CAD build for the part. Positions are in the model's coordinates, mm. Coordinates: 2 decimals unless noted, no trailing zeros. Loops run counter-clockwise (first coordinate to the right, second up) from the corner with the lowest first, then second, coordinate; pieces in that order, holes last. Notation, with made-up numbers: (83.5, 76) - (109.5, 76) arc R22 cw to (109.5, 92) - close; hole circle Ø9 at (49.25, 30). An arc over 180 degrees is marked (long way). Put each result on its own line as item: value.
```python
from build123d import *

# Parameters (mm, degrees)
SKETCH_1_W          = 23.5
SKETCH_1_H          = 10
SKETCH_1_R          = 1.6
EXTRUDE_1_DEPTH     = 5
SKETCH_2_R          = 2
CUT_EXTRUDE_1_DEPTH = 10


with BuildPart() as part:
    # 草图1 → 凸台-拉伸1 (new body)
    with BuildSketch(Plane.XY):
        Rectangle(SKETCH_1_W, SKETCH_1_H)
        with Locations((-8.5, 0)):
            Circle(SKETCH_1_R, mode=Mode.SUBTRACT)
        with Locations((8.5, 0)):
            Circle(SKETCH_1_R, mode=Mode.SUBTRACT)
    extrude(amount=EXTRUDE_1_DEPTH)

    # 草图2 → 切除-拉伸1 (cut)
    with BuildSketch(Plane.XY.offset(5)):
        Circle(SKETCH_2_R)
    extrude(amount=-CUT_EXTRUDE_1_DEPTH, mode=Mode.SUBTRACT)


solid = part.part
```
Q1. Wall check: L1, parallel to X at y = -0.5, z = 2.15; L2, parallel to Y at x = 8.5, z = 1.4; L3, parallel to Y at x = 0, z = 1.6. Give the ranges that are in metal, low to high. Write a range as from..to.
Determined:
L1: -11.75..-10.02, -6.98..-1.94, 1.94..6.98, 10.02..11.75
L2: -5..-1.6, 1.6..5
L3: -5..-2, 2..5
Q2. Slice it at B-B, the plane z = 4. Give the cut face in (x, y), then the cut area to 3 significant figures.
Determined:
outline: (-11.75, -5) - (11.75, -5) - (11.75, 5) - (-11.75, 5) - close; hole circle Ø3.2 at (-8.5, 0); hole circle Ø4 at (0, 0); hole circle Ø3.2 at (8.5, 0)
area: 206 mm2
Q3. Slice it at C-C, the plane x = -8.5. Give the cut face in (y, z).
Determined:
outline: (-5, 0) - (-1.6, 0) - (-1.6, 5) - (-5, 5) - close; (1.6, 0) - (5, 0) - (5, 5) - (1.6, 5) - close
Q4. Slice it at A-A, the plane x = 0. Give the cut face in (y, z), then the cut area to 3 significant figures.
Determined:
outline: (-5, 0) - (-2, 0) - (-2, 5) - (-5, 5) - close; (2, 0) - (5, 0) - (5, 5) - (2, 5) - close
area: 30.0 mm2
Q5. Mould opens along X. For faces 1 (the flat face through (0, 5, 2)), 2 (the flat face through (11.75, 0, 2)), 3 (the cylindrical face through (-10.1, 0.07, 2.46)), 4 (the flat face through (-11.75, 0, 2)) say: +X half, -X half, draft (parallel to the pull), parting line (faces both ways), or undercut.
Determined:
face 1: draft
face 2: +X half
face 3: undercut
face 4: -X half
